Design review of the part built by this model. Coordinates are the model's own, in mm. Face numbers are marked on the shaded views. A direction names the side the tool comes from. Give positions to 0.01 mm unless a question says otherwise; leave off trailing zeros. Loops run counter-clockwise (first coordinate to the right, second up) from the corner with the lowest first, then second, coordinate; pieces in that order, holes last. Notation, with made-up numbers: (76, -29.5) -> (117, -29.5) arc R21 ccw to (117, -1.5) -> close; hole circle Ø4 at (35.25, 33). An arc over 180 degrees is marked (long way). Use a Markdown table: item, result. Add a question column.
1. Add section B-B (y = 89). State the section outline as (x, z) points, and give its area (3 significant figures).
2. Add section A-A (y = 107). State the section outline as (x, z) points.
3. For the marked faces 1, 2 and 3, list the 3-axis set-ups (+Z, -Z, +X, -X, +Y, -Y) from which the entire face can be reached by the end or side of a thin tool; tool diameter is ignored.
4. Add section D-D (y = 49.5). State the section outline as (x, z) points, and give its area (3 significant figures).
5. Add section C-C (x = 0). Count the separate pieces of the cut face and the enclosed holes in it, and give its area (3 significant figures).
6. To check wall thickness, follow line 1 (Y direction, x = 0, z = 1.75); line 2 (Y direction, x = 0, z = -5.55); line 3 (Y direction, x = -35.5, z = -8.5). State the ranges of each line that lie inside material, in increasing order.
7. Draft analysis for pull direction Y (two halves, no side actions). For the marked faces 4, 5, 6 and 7, state which applies: pulls with the +Y half, pulls with the -Y half, needs draft (parallel to the pull), parting line crosses it, or undercut.
8. For pin 1 Ø6.5 at (x, y) = (-31.18, 107) entering from -Z; pin 2 Ø2 at (x, y) = (26, 35) entering from +Z; pin 3 Ø2 at (x, z) = (1, -9.5) entering from +Y; pin 4 Ø9.5 at (x, y) = (0, 161) entering from -Z, all flat-tipped, find the tip position at first contact; note any pin that passes through.
```python
from build123d import *

# Parameters (mm, degrees)
SKETCH1_R                         = 8
BOSS_EXTRUDE1_DEPTH               = 10
SKETCH2_R                         = 12.5
CUT_EXTRUDE1_DEPTH                = 10
SKETCH3_R                         = 3.5
CUT_EXTRUDE2_DEPTH                = 21
SKETCH4_R                         = 6
CUT_EXTRUDE3_DEPTH                = 6
CIRPATTERN1_COUNT                 = 6
TAP_DRILL_FOR_M10X1_25_TAP2_D     = 8.8
TAP_DRILL_FOR_M10X1_25_TAP2_DEPTH = 24
TAP_DRILL_FOR_M10X1_25_TAP2_TIP   = 2.643786724
CUT_EXTRUDE4_DEPTH                = 4
FILLET1_R                         = 2
FILLET1_OF_MIRROR1_R              = 2


with BuildPart() as part:
    # Sketch1 → Boss-Extrude1 (new body, symmetric)
    with BuildSketch(Plane.XY):
        with BuildLine():
            Line((46, 125), (46, 0))
            Line((46, 0), (-46, 0))
            Line((-46, 0), (-46, 125))
            ThreePointArc((-46, 125), (0, 171), (46, 125))
        make_face()
        with Locations((0, 125)):
            Circle(SKETCH1_R, mode=Mode.SUBTRACT)
    extrude(amount=BOSS_EXTRUDE1_DEPTH, both=True)

    # Sketch2 → Cut-Extrude1 (cut)
    with BuildSketch(Plane.XY.offset(10)):
        with Locations((0, 125)):
            Circle(SKETCH2_R)
    extrude(amount=-CUT_EXTRUDE1_DEPTH, mode=Mode.SUBTRACT)

    # Sketch3 → Cut-Extrude2 (cut, through all)
    with BuildSketch(Plane.XY.offset(10)):
        with Locations((0, 161)):
            Circle(SKETCH3_R)
    cut_extrude2 = extrude(amount=-CUT_EXTRUDE2_DEPTH, mode=Mode.SUBTRACT)

    # Sketch4 → Cut-Extrude3 (cut)
    with BuildSketch(Plane(origin=(0, 0, -10), x_dir=(-1, 0, 0), z_dir=(0, 0, -1))):
        with Locations((0, 161)):
            Circle(SKETCH4_R)
    cut_extrude3 = extrude(amount=-CUT_EXTRUDE3_DEPTH, mode=Mode.SUBTRACT)

    # CirPattern1: Cut-Extrude2, Cut-Extrude3 ×6 about axis
    cirpattern1_axis = Axis((0, 125, 0), (0, 0, 1))
    for i in range(1, CIRPATTERN1_COUNT):
        add(cut_extrude2.rotate(cirpattern1_axis, i * 360 / CIRPATTERN1_COUNT), mode=Mode.SUBTRACT)
        add(cut_extrude3.rotate(cirpattern1_axis, i * 360 / CIRPATTERN1_COUNT), mode=Mode.SUBTRACT)

    # Tap Drill for M10x1.25 Tap2
    with Locations(Plane(origin=(0, 0, 0), x_dir=(-1, 0, 0), z_dir=(0, -1, 0))):
        with Locations((30, 0), (-30, 0)):
            Hole(TAP_DRILL_FOR_M10X1_25_TAP2_D / 2, depth=TAP_DRILL_FOR_M10X1_25_TAP2_DEPTH)
            with Locations((0, 0, -(TAP_DRILL_FOR_M10X1_25_TAP2_DEPTH + TAP_DRILL_FOR_M10X1_25_TAP2_TIP / 2))):  # 118° drill point
                Cone(0, TAP_DRILL_FOR_M10X1_25_TAP2_D / 2, TAP_DRILL_FOR_M10X1_25_TAP2_TIP, mode=Mode.SUBTRACT)

    # Sketch11 → Cut-Extrude4 (cut)
    with BuildSketch(Plane.XY.offset(10)):
        with BuildLine():
            Line((-34, 74.206299603), (-34, 12))
            Line((-34, 12), (34, 12))
            Line((34, 12), (34, 74.206299603))
            ThreePointArc((34, 74.206299603), (31.051285766, 79.372502771), (25.103448276, 79.460820334))
            ThreePointArc((25.103448276, 79.460820334), (0, 73), (-25.103448276, 79.460820334))
            ThreePointArc((-25.103448276, 79.460820334), (-31.051285766, 79.372502771), (-34, 74.206299603))
        make_face()
    cut_extrude4 = extrude(amount=-CUT_EXTRUDE4_DEPTH, mode=Mode.SUBTRACT)

    # Fillet1
    fillet1_edges = [part.edges().sort_by_distance(p)[0] for p in [
        (31.051285766, 79.372502771, 6),
        (34, 43.103149802, 6),
        (0, 12, 6),
        (-34, 43.103149802, 6),
        (-31.051285766, 79.372502771, 6),
        (0, 73, 6),
    ]]
    fillet(fillet1_edges, radius=FILLET1_R)

    # Mirror1: Cut-Extrude4 across plane
    add(cut_extrude4.mirror(Plane.XY), mode=Mode.SUBTRACT)

    # Fillet1 of Mirror1
    fillet1_of_mirror1_edges = [part.edges().sort_by_distance(p)[0] for p in [
        (31.051285766, 79.372502771, -6),
        (34, 43.103149802, -6),
        (0, 12, -6),
        (-34, 43.103149802, -6),
        (-31.051285766, 79.372502771, -6),
        (0, 73, -6),
    ]]
    fillet(fillet1_of_mirror1_edges, radius=FILLET1_OF_MIRROR1_R)


solid = part.part
```
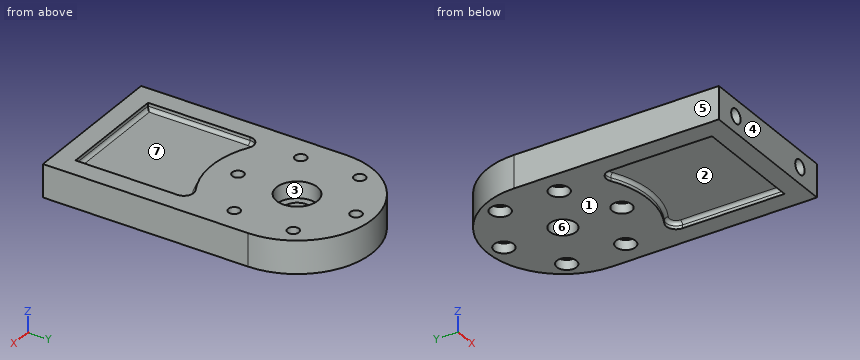
Taken from the geometry:
| question | item | result |
|---|---|---|
| 1 | outline | (-46, -10) -> (-6, -10) -> (-6, -4) -> (-3.5, -4) -> (-3.5, 10) -> (-46, 10) -> close; (3.5, -4) -> (6, -4) -> (6, -10) -> (46, -10) -> (46, 10) -> (3.5, 10) -> close |
| 1 | area | 1,670 mm^2 |
| 2 | outline | (-46, -10) -> (-37.18, -10) -> (-37.18, -4) -> (-34.68, -4) -> (-34.68, 10) -> (-46, 10) -> close; (-27.68, -4) -> (-25.18, -4) -> (-25.18, -10) -> (25.18, -10) -> (25.18, -4) -> (27.68, -4) -> (27.68, 10) -> (-27.68, 10) -> close; (34.68, -4) -> (37.18, -4) -> (37.18, -10) -> (46, -10) -> (46, 10) -> (34.68, 10) -> close |
| 3 | face 1 | -Z, +X, -X, +Y, -Y |
| 3 | face 2 | -Z |
| 3 | face 3 | +Z |
| 4 | outline | (-46, -10) -> (-34, -10) -> (-34, -8) arc R2 cw to (-32, -6) -> (32, -6) arc R2 cw to (34, -8) -> (34, -10) -> (46, -10) -> (46, 10) -> (34, 10) -> (34, 8) arc R2 cw to (32, 6) -> (-32, 6) arc R2 cw to (-34, 8) -> (-34, 10) -> (-46, 10) -> close |
| 4 | area | 1,300 mm^2 |
| 5 | separate pieces | 4 |
| 5 | enclosed holes | 0 |
| 5 | area | 2,190 mm^2 |
| 6 | line 1 | y = 0 to 85.5, 92.5 to 112.5, 137.5 to 157.5, 164.5 to 171 |
| 6 | line 2 | y = 0 to 83, 95 to 117, 133 to 155, 167 to 171 |
| 6 | line 3 | y = 0 to 102.84, 111.16 to 138.84, 147.16 to 154.25 |
| 7 | face 4 | pulls with the -Y half |
| 7 | face 5 | needs draft |
| 7 | face 6 | undercut |
| 7 | face 7 | undercut |
| 8 | pin 1 | passes through |
| 8 | pin 2 | stops at z = 6 |
| 8 | pin 3 | stops at y = 171 |
| 8 | pin 4 | stops at z = -4 |
